Answer from the drawing. Dimensions are ordinates in mm from the lowest x, y and z of the part. A direction names the side the tool comes from. Give positions to 0.01 mm unless a question says otherwise; leave off trailing zeros. Order: outer loops, then holes, each group sorted by start corner. A loop starts at its lowest first (then second) coordinate and runs counter-clockwise, first axis right, second up.
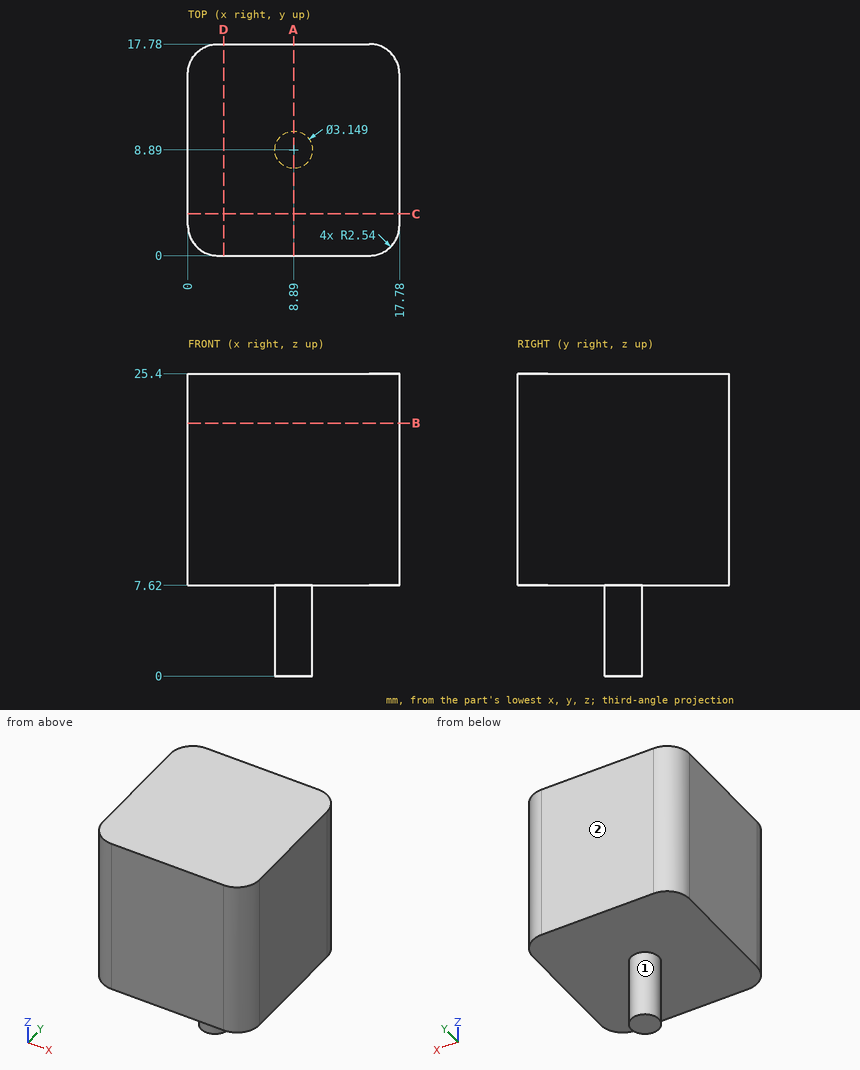
1. The part is cut by section C-C (y = 3.5). Write down the section's boundary in (x, z), then the cut area to 3 significant figures.
Findings below:
outline: (0, 7.62) - (17.78, 7.62) - (17.78, 25.4) - (0, 25.4) - close
area: 316 mm2
2. Which of the six approach directions +Z, -Z, +X, -X, +Y, -Y give full straight-line access (tool end or side, diameter ignored) to the marked faces 1 and 2?
Findings below:
face 1: -Z
face 2: +Z, -Z, +X, -X, +Y
3. Straight lines are drawn through the part: probe 1 along Z at (x, y) = (6.5, 10.75); probe 2 along Y at (x, z) = (1.25, 12); probe 3 along X at (y, z) = (7.75, 6.25). For each, find the intervals that lie inside material, in ascending order.
Findings below:
probe 1: z = 7.62 to 25.4
probe 2: y = 0.35 to 17.43
probe 3: x = 7.8 to 9.98
4. The part is cut by section B-B (z = 21.25). Write down the section's boundary in (x, y), then the cut area to 3 significant figures.
Findings below:
outline: (0, 2.54) arc R2.54 ccw to (2.54, 0) - (15.24, 0) arc R2.54 ccw to (17.78, 2.54) - (17.78, 15.24) arc R2.54 ccw to (15.24, 17.78) - (2.54, 17.78) arc R2.54 ccw to (0, 15.24) - close
area: 311 mm2
5. The part is cut by section A-A (x = 8.89). Write down the section's boundary in (y, z).
Findings below:
outline: (0, 7.62) - (7.32, 7.62) - (7.32, 0) - (10.46, 0) - (10.46, 7.62) - (17.78, 7.62) - (17.78, 25.4) - (0, 25.4) - close
6. Given P1, Ø3, axis at x = 5, z = 19, coming from the -Y side; P2, Ø3, axis at x = 7, z = 4, coming from the -Y side, each flat-ended and moving along its own axis, determine where each tip first touches the part or whether it passes through.
Findings below:
P1: stops at y = 0
P2: stops at y = 7.36
